The listing builds one solid part. Answer for the finished solid, in the listing's coordinates (mm). Coordinates: 2 decimals unless noted, no trailing zeros. Write each loop counter-clockwise with the first axis right and the second up, starting at its lowest first coordinate (ties: lowest second). Pieces come first, ordered by that corner, then holes. Notation, with made-up numbers: M -28.5,79 L 5.5,79 A13 ccw 5.5,101 Z; hole C 3,51.25 d2. An arc over 180 degrees is marked long. Put each result on its own line as item: value. Start each with the question number.
```python
from build123d import *

# Parameters (mm, degrees)
SKETCH3_R           = 3
SKETCH3_R_2         = 1
SKETCH3_R_3         = 1.500000001
BOSS_EXTRUDE1_DEPTH = 1.5875


with BuildPart() as part:
    # Sketch3 → Boss-Extrude1 (new body)
    with BuildSketch(Plane.XY):
        with BuildLine():
            Line((-11.499999999, 31.641209076), (19.500000007, 31.641209076))
            ThreePointArc((19.500000007, 31.641209076), (22.500000018, 28.641209065), (19.500000007, 25.641209053))
            Line((19.500000007, 25.641209053), (19.289245586, 25.641209053))
            Line((19.289245586, 25.641209053), (6.042590494, -4.911559932))
            ThreePointArc((6.042590494, -4.911559932), (6.937456234, -7.718176584), (5, -9.937218057))
            Line((5, -9.937218057), (5, -20.212517806))
            ThreePointArc((5, -20.212517806), (8.217909302, -23.031803227), (7.623388784, -27.268530255))
            Line((7.623388784, -27.268530255), (13.255537043, -33.795798194))
            ThreePointArc((13.255537043, -33.795798194), (15.860860714, -36.911906153), (11.799598856, -36.975091304))
            Line((11.799598856, -36.975091304), (-3.799598854, -36.975091304))
            ThreePointArc((-3.799598854, -36.975091304), (-7.037028015, -37.86441568), (-7.553929711, -34.547088736))
            Line((-7.553929711, -34.547088736), (-13.250643923, -21.881287835))
            ThreePointArc((-13.250643923, -21.881287835), (-14.64398835, -20.503360892), (-13.885312196, -18.696567642))
            Line((-13.885312196, -18.696567642), (-12.58228364, 25.843234412))
            ThreePointArc((-12.58228364, 25.843234412), (-14.449061209, 29.191697969), (-11.499999999, 31.641209076))
        make_face()
        with Locations((4, -24.6)):
            Circle(SKETCH3_R, mode=Mode.SUBTRACT)
        with Locations((-12.927736724, -20.161336981)):
            Circle(SKETCH3_R_2, mode=Mode.SUBTRACT)
        with Locations((4, -7.108790933)):
            Circle(SKETCH3_R_3, mode=Mode.SUBTRACT)
        with Locations((-5.815163291, -35.975091304)):
            Circle(SKETCH3_R_2, mode=Mode.SUBTRACT)
        with Locations((13.815163293, -35.975091304)):
            Circle(SKETCH3_R_2, mode=Mode.SUBTRACT)
        with Locations((-11.499999999, 28.641209067)):
            Circle(SKETCH3_R_2, mode=Mode.SUBTRACT)
        with Locations((4, 28.641209067)):
            Circle(SKETCH3_R_2, mode=Mode.SUBTRACT)
        with Locations((19.500000007, 28.641209065)):
            Circle(SKETCH3_R_2, mode=Mode.SUBTRACT)
        Polygon((-9.109355809, 25.641209053), (3, 25.641209053), (3, -2.288434183), align=None, mode=Mode.SUBTRACT)
        with BuildLine():
            Line((5.500000007, 30.641209065), (5.500000007, 26.641209065))
            Line((5.500000007, 26.641209065), (16.612506499, 26.612956076))
            ThreePointArc((16.612506499, 26.612956076), (15.971383713, 28.624004515), (16.59286586, 30.641209065))
            Line((16.59286586, 30.641209065), (5.500000007, 30.641209065))
        make_face(mode=Mode.SUBTRACT)
        with BuildLine():
            Line((2.500000001, 30.641209067), (-8.592865852, 30.641209067))
            ThreePointArc((-8.592865852, 30.641209067), (-7.971383705, 28.624004518), (-8.612506491, 26.612956078))
            Line((-8.612506491, 26.612956078), (2.500000001, 26.641209067))
            Line((2.500000001, 26.641209067), (2.500000001, 30.641209067))
        make_face(mode=Mode.SUBTRACT)
        with BuildLine():
            Line((3, -20.212517806), (3, -9.937218057))
            ThreePointArc((3, -9.937218057), (2.676302312, -9.800969313), (2.370745742, -9.627824589))
            Line((2.370745742, -9.627824589), (-10.705156103, -19.710319003))
            Line((-10.705156103, -19.710319003), (0.009629689, -22.519869047))
            ThreePointArc((0.009629689, -22.519869047), (1.251015388, -21.03726459), (3, -20.212517806))
        make_face(mode=Mode.SUBTRACT)
        Polygon((5, 25.641209053), (17.109355816, 25.641209053), (5, -2.288434184), align=None, mode=Mode.SUBTRACT)
        with BuildLine():
            Line((1.149490439, -8.043988902), (-11.866425305, -18.080229562))
            Line((-11.866425305, -18.080229562), (-10.631706445, 24.124626881))
            Line((-10.631706445, 24.124626881), (1.957409506, -4.911559931))
            ThreePointArc((1.957409506, -4.911559931), (1.095067152, -6.359547882), (1.149490439, -8.043988902))
        make_face(mode=Mode.SUBTRACT)
        with BuildLine():
            Line((-3.631490152, -34.975091304), (11.631490154, -34.975091304))
            Line((11.631490154, -34.975091304), (6.109164807, -28.575100479))
            ThreePointArc((6.109164807, -28.575100479), (4, -29.1), (1.890835193, -28.575100479))
            Line((1.890835193, -28.575100479), (-3.631490152, -34.975091304))
        make_face(mode=Mode.SUBTRACT)
        with BuildLine():
            Line((-11.157493782, -21.659322937), (-0.497646084, -24.454467529))
            ThreePointArc((-0.497646084, -24.454467529), (-0.297387472, -25.935088354), (0.376611216, -27.268530255))
            Line((0.376611216, -27.268530255), (-5.255537041, -33.795798194))
            ThreePointArc((-5.255537041, -33.795798194), (-5.490888453, -33.748581518), (-5.729930654, -33.72670624))
            Line((-5.729930654, -33.72670624), (-11.157493782, -21.659322937))
        make_face(mode=Mode.SUBTRACT)
    extrude(amount=BOSS_EXTRUDE1_DEPTH)


solid = part.part
```
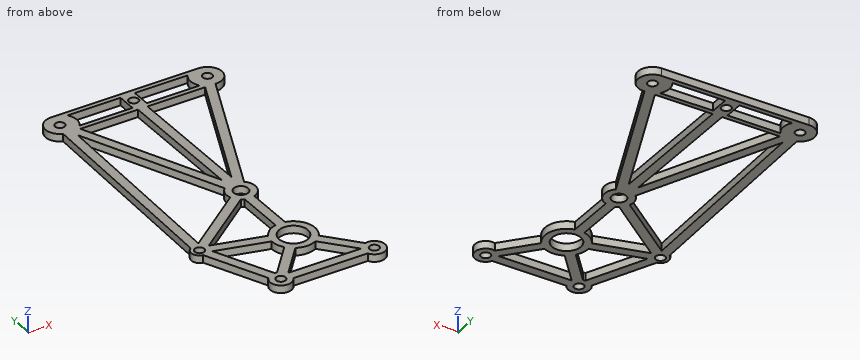
1) A cutting plane is placed at A-A on x = 4. Write down the section's boundary in (y, z), then the cut area to 3 significant figures.
2) A cutting plane is placed at D-D on z = 0.9. State how many separate pieces and enclosed holes the cut face has, then the cut area to 3 significant figures.
3) Straight lines are drawn through the part: probe 1 along Y at (x, z) = (4, 1.1); probe 2 along Y at (x, z) = (6, 1); probe 3 along Y at (x, z) = (8, 1.55) (3 decimals). For each, find the intervals that lie inside material, in ascending order.
4) A cutting plane is placed at B-B on y = -3. Write down the section's boundary in (x, z), then the cut area to 3 significant figures.
5) Given pin 1 Ø0.5 at (x, z) = (-3.5, 0.5) entering from -Y; pin 2 Ø0.5 at (y, z) = (29.5, 1) entering from +X, each flat-ended and moving along its own axis, determine where each tip first touches the part or whether it passes through.
6) A cutting plane is placed at C-C on x = 14. Write down the section's boundary in (y, z), then the cut area to 3 significant figures.
Answers follow:
1. outline: M -36.98,0 L -34.98,0 L -34.98,1.59 L -36.98,1.59 Z; M -29.1,0 L -27.6,0 L -27.6,1.59 L -29.1,1.59 Z; M -21.6,0 L -8.61,0 L -8.61,1.59 L -21.6,1.59 Z; M -5.61,0 L 27.64,0 L 27.64,1.59 L -5.61,1.59 Z; M 29.64,0 L 31.64,0 L 31.64,1.59 L 29.64,1.59 Z
1. area: 82.1 mm²
2. separate pieces: 1
2. enclosed holes: 16
2. area: 652 mm²
3. probe 1: y = -36.98 to -34.98, -29.1 to -27.6, -21.6 to -8.61, -5.61 to 27.64, 29.64 to 31.64
3. probe 2: y = -36.98 to -34.98, -28.63 to -26.84, -22.36 to -20.57, -9.34 to 0.02, 25.64 to 26.64, 30.64 to 31.64
3. probe 3: y = -36.975 to -34.975, -30.766 to -27.705, -26.662 to -22.538, -0.397 to 4.631, 25.641 to 26.635, 30.641 to 31.641
4. outline: M -13.43,0 L -11.43,0 L -11.43,1.59 L -13.43,1.59 Z; M 1.13,0 L 6.87,0 L 6.87,1.59 L 1.13,1.59 Z
4. area: 12.3 mm²
5. pin 1: stops at y = -36.98
5. pin 2: stops at x = 22.44
6. outline: M -38.22,0 L -36.96,0 L -36.96,1.59 L -38.22,1.59 Z; M -34.99,0 L -33.73,0 L -33.73,1.59 L -34.99,1.59 Z; M 13.44,0 L 18.47,0 L 18.47,1.59 L 13.44,1.59 Z; M 25.64,0 L 26.62,0 L 26.62,1.59 L 25.64,1.59 Z; M 30.64,0 L 31.64,0 L 31.64,1.59 L 30.64,1.59 Z
6. area: 15.1 mm²
